Solid Edge part; units mm, degrees
sketch "Sketch1" plane through (0, 0, 0) normal (0, -1, 0) x (1, 0, 0)
  line L0 (187.1606, 27.9036) -> (-320.8394, 27.9036)
  line L1 (-320.8394, 27.9036) -> (-320.8394, 15.2036)
  line L2 (-320.8394, 15.2036) -> (187.1606, 15.2036)
  line L3 (187.1606, 15.2036) -> (187.1606, 27.9036)
extrude "Protrusion1" add sketch "Sketch1" against normal blind 12.7
sketch "Sketch2" plane through (-320.8394, 6.35, 21.5536) normal (-1, 0, 0) x (0, -1, 0)
  line L0 (6.35, 6.35) -> (-8.336, 21.036)
  arc A0 (-8.336, 21.036) -> (-16.2414, 24.3105) centre (-16.2414, 13.1305) ccw
  line L1 (-16.2414, 24.3105) -> (-17.9544, 24.3105)
  line L2 (-17.9544, 24.3105) -> (-17.9544, -6.35)
  line L3 (-17.9544, -6.35) -> (-6.35, -6.35)
extrude "ExtrudedProtrusion_2" add sketch "Sketch2" against normal blind 12.7 material side at (-320.8394, 7.3784, 35.2112)
sketch "Sketch3" plane through (187.1606, 6.35, 21.5536) normal (1, 0, 0) x (0, 1, 0)
  line L0 (8.336, 21.036) -> (-6.35, 6.35)
  line L1 (-6.35, 6.35) -> (-6.35, -6.35)
  line L2 (-6.35, -6.35) -> (17.9544, -6.35)
  line L3 (17.9544, -6.35) -> (17.9544, 23.4399)
  line L4 (17.9544, 23.4399) -> (17.9544, 24.3105)
  line L5 (17.9544, 24.3105) -> (14.1772, 24.3105)
  arc A0 (14.1772, 24.3105) -> (9.5809, 22.3419) centre (14.1772, 17.9605) ccw
  line L6 (9.5809, 22.3419) -> (8.336, 21.036)
extrude "ExtrudedProtrusion_3" add sketch "Sketch3" against normal blind 12.7
hole "Hole_1" at (180.8106, 24.3044, 39.5141) direction (0, -1, 0) diameter 6.35 end up to next
hole "Hole1" at (180.8106, 24.3044, 21.5536) direction (0, -1, 0) diameter 6.35 end up to next
hole "Hole_3" at (-314.4894, 24.3044, 39.5141) direction (0, -1, 0) diameter 6.35 end up to next
hole "Hole2" at (-314.4894, 24.3044, 21.5536) direction (0, -1, 0) diameter 6.35 end up to next
fillet "Round_1" radius 6.35 4 edges at (-66.8394, 0, 27.9036) (-66.8394, 12.7, 27.9036) (-66.8394, 0, 15.2036) (-66.8394, 12.7, 15.2036)
Read the model definition and answer for the solid it produces. Units are mm, in the model's axes. A direction names the side the tool comes from. Give positions to 0.01 mm unless a question says otherwise; leave off trailing zeros. Answer in a Markdown table with one row per item. Add a question column.
Item 1: Determine the mould class of faces 4 (the face through (-315, 24.304, 31)), 5 (the face through (-320.839, 15, 27)), 6 (the face through (174.461, 17, 30)) for opening direction X: pulls with the +X half, pulls with the -X half, needs draft (parallel to the pull), parting line crosses it, or undercut.
Item 2: Flat-ended cylindrical pins translate along their axes: P1, Ø12, axis at x = -253, z = 25.5, coming from the +Y side; P2, Ø5.5, axis at x = 180.81, z = 39.51, coming from the -Y side; P3, Ø8.5, axis at x = -314.49, z = 39.51, coming from the -Y side; P4, Ø8, axis at x = -135, y = 11, coming from the +Z side. Find the tip coordinate at first contact, or state that the pin passes through.
Item 3: A tool of negligible diameter and unlimited length cuts with its end or side. For faces 1 (the face through (-63.283, 1.714, 17.214)), 2 (the face through (181, 24.304, 30)), 3 (the face through (-314.58, 18.26, 44.99)), from which of +Z, -Z, +X, -X, +Y, -Y can it reach the whole face along a straight path? Write none if from no direction.
Item 4: Find the intervals of material crossed by L1, parallel to X at y = 4.5, z = 21; L2, parallel to X at y = 20.5, z = 26.5; L3, parallel to X at y = 20, z = 23, in increasing order.
Recorded:
| question | item | result |
|---|---|---|
| 1 | face 4 | needs draft |
| 1 | face 5 | pulls with the -X half |
| 1 | face 6 | undercut |
| 2 | P1 | stops at y = 12.7 |
| 2 | P2 | passes through |
| 2 | P3 | stops at y = 7.36 |
| 2 | P4 | stops at z = 27.87 |
| 3 | face 1 | none |
| 3 | face 2 | +Z, -Z, +X, -X, +Y |
| 3 | face 3 | +Z, -X, -Y |
| 4 | L1 | x = -320.84 to -317.62, -311.36 to 177.68, 183.94 to 187.16 |
| 4 | L2 | x = -320.84 to -308.14, 174.46 to 187.16 |
| 4 | L3 | x = -320.84 to -317.32, -311.66 to -308.14, 174.46 to 177.98, 183.64 to 187.16 |
